Autodesk Fusion 360 part; units mm, degrees
sketch "Name Sign LED Holder Top" plane through (0, 0, 0) normal (0, 1, 0) x (1, 0, 0)
  line L0 (0.5771, -64.3591) -> (5.5771, -64.3591)
  line L1 (5.5771, -64.3591) -> (5.5771, -28.5209)
  line L2 (5.5771, -28.5209) -> (36.754, -15.7343)
  line L3 (36.754, -15.7343) -> (32.9594, -6.4822)
  line L4 (32.9594, -6.4822) -> (0.5771, -19.7631)
  line L5 (0.5771, -19.7631) -> (0.5771, -64.3591)
  line L6 (0.5771, -64.3591) -> (5.5771, -62.3085)
  line L7 (32.9594, -6.4822) -> (32.9594, -17.2905)
  dimension "d1" = 5
  dimension "d2" = 10
  dimension "d3" = 112.3
  dimension "d16" = 44.596
  dimension "d18" = 22.3
  dimension "d20" = 35
extrude "Extrude1" add sketch "Name Sign LED Holder Top" along normal blind 220 contours L1 L2 L4 L5 L6 L7
sketch "LED Grooves" plane through (0.5771, 0, 0) normal (-1, 0, 0) x (0, -1, 0)
  line L0 (0, 19.7631) -> (0, 64.3591)
  line L1 (-220, 64.3591) -> (-220, 19.7631)
  line L2 (-220, 19.7631) -> (0, 19.7631)
  line L3 (-215, 62.3591) -> (-5, 62.3591)
  line L4 (-5, 62.3591) -> (-5, 52.3591)
  line L5 (-5, 52.3591) -> (-215, 52.3591)
  line L6 (-215, 52.3591) -> (-215, 62.3591)
  line L7 (-215, 48.3591) -> (-5, 48.3591)
  line L8 (-5, 48.3591) -> (-5, 38.3591)
  line L9 (-5, 38.3591) -> (-215, 38.3591)
  line L10 (-215, 38.3591) -> (-215, 48.3591)
  line L11 (-5, 62.3591) -> (-15, 62.3591)
  line L12 (-15, 52.3591) -> (-5, 52.3591)
  line L13 (-5, 52.3591) -> (-5, 62.3591)
  line L14 (-5, 48.3591) -> (-15, 48.3591)
  line L15 (-15, 38.3591) -> (-5, 38.3591)
  line L16 (-5, 38.3591) -> (-5, 48.3591)
  line L17 (0, 64.3591) -> (-220, 64.3591)
  dimension "d6" = 210
  dimension "d7" = 210
  dimension "d8" = 5
  dimension "d9" = 5
  dimension "d12" = 10
  dimension "d13" = 10
  dimension "d22" = 4
  dimension "d30" = 2
extrude "Extrude2" cut sketch "LED Grooves" against normal blind 3 contours L3 L4 L5 L6 L11 L12 L13 | L7 L8 L9 L10 L14 L15 L16
sketch "Top LED Hole" plane through (3.5771, 0, 0) normal (-1, 0, 0) x (0, -1, 0)
  line L0 (-215, 52.3591) -> (-5, 52.3591)
  line L1 (-5, 52.3591) -> (-5, 62.3591)
  line L2 (-5, 62.3591) -> (-215, 62.3591)
  line L3 (-215, 62.3591) -> (-215, 52.3591)
  line L4 (-5, 62.3591) -> (-15, 62.3591)
  line L5 (-15, 62.3591) -> (-15, 52.3591)
  line L6 (-15, 52.3591) -> (-5, 52.3591)
  line L7 (-5, 52.3591) -> (-5, 62.3591)
  dimension "d33" = 10
  dimension "d34" = 10
sketch "Bottom LED Hole" plane through (3.5771, 0, 0) normal (-1, 0, 0) x (0, -1, 0)
  line L0 (-215, 38.3591) -> (-5, 38.3591)
  line L1 (-5, 38.3591) -> (-5, 48.3591)
  line L2 (-215, 48.3591) -> (-215, 38.3591)
  line L3 (-5, 48.3591) -> (-15, 48.3591)
  line L4 (-15, 48.3591) -> (-15, 38.3591)
  line L5 (-15, 38.3591) -> (-5, 38.3591)
  line L6 (-5, 38.3591) -> (-5, 48.3591)
  line L7 (-5, 48.3591) -> (-215, 48.3591)
  dimension "d26" = 10
  dimension "d27" = 10
extrude "Extrude3" cut sketch "Top LED Hole" sketch "Bottom LED Hole" against normal blind 2 contours L0 L1 L2 L4 L5 L6 L7 of sketch 2 contours L0 L1 L3 L4 L5 L6 L7
sketch "Magnet Holes" plane through (7.0215, 0, 17.1201) normal (-0.3795, 0, -0.9252) x (0, -1, 0)
  line L0 (0, -28.0347) -> (0, 6.9653)
  line L1 (0, 6.9653) -> (-220, 6.9653)
  line L2 (-220, 6.9653) -> (-220, -28.0347)
  line L3 (-220, -28.0347) -> (0, -28.0347)
  circle A0 centre (-210, -5.5347) radius 2.75
  dimension "d39" = 5.5
  dimension "d47" = 10
  dimension "d48" = 12.5
extrude "Extrude4" cut sketch "Magnet Holes" against normal blind 1.5 contours A0
pattern_linear "R-Pattern1" count 4 spacing 66.6667 along (0, -1, 0) count 2 spacing 15 along (0.9252, 0, -0.3795) of "Extrude4"
equation "d4 = 200 mm + 10 mm + 5 mm + 5 mm"
equation "d6 = 200 mm + 10 mm"
equation "d7 = 200 mm + 10 mm"
equation "d16 = 50 mm - 5.404 mm"
equation "magnet_hole_diameter = 5.5 mm"
equation "magnet_hole_depth = 1.5 mm"
equation "d39 = magnet_hole_diameter"
equation "d45 = magnet_pattern_height"
equation "magnet_hole_side_offset = 10 mm"
equation "d47 = magnet_hole_side_offset"
equation "d48 = vertical_part_width + magnet_hole_top_offset"
equation "magnet_hole_top_offset = 7.5 mm"
equation "magnet_pattern_length = 220.00 mm - 2 * ( magnet_hole_side_offset )"
equation "magnet_pattern_height = 35.00 mm - vertical_part_width - 2 * ( magnet_hole_top_offset )"
equation "vertical_part_width = 5.00 mm"
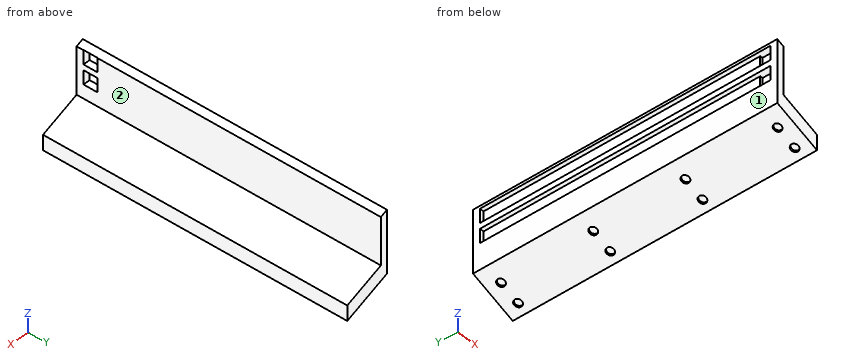
The listing builds one solid part. Answer for the finished solid, in the listing's coordinates (mm). Face numbers are marked on the shaded views. A direction names the side the tool comes from. Give positions to 0.01 mm unless a question says otherwise; leave off trailing zeros. Loops run counter-clockwise (first coordinate to the right, second up) from the corner with the lowest first, then second, coordinate; pieces in that order, holes last.
Item 1: A cutting plane is placed at C-C (y = 144). Give the vertices of the cut face in (x, z) (1 decimal).
Derived:
outline: (0.6, 19.8) - (9.7, 16) - (10.2, 17.4) - (15.2, 15.4) - (14.6, 14) - (23.6, 10.3) - (24.1, 11.7) - (29.1, 9.7) - (28.5, 8.3) - (33, 6.5) - (33, 17.3) - (5.6, 28.5) - (5.6, 62.3) - (0.6, 64.4) - (0.6, 62.4) - (3.6, 62.4) - (3.6, 52.4) - (0.6, 52.4) - (0.6, 48.4) - (3.6, 48.4) - (3.6, 38.4) - (0.6, 38.4) - close
Item 2: A cutting plane is placed at B-B (y = 31.5). Give the vertices of the cut face in (x, z), then the cut area to 3 significant figures.
Derived:
outline: (0.58, 19.76) - (32.96, 6.48) - (32.96, 17.29) - (5.58, 28.52) - (5.58, 62.31) - (0.58, 64.36) - (0.58, 62.36) - (3.58, 62.36) - (3.58, 52.36) - (0.58, 52.36) - (0.58, 48.36) - (3.58, 48.36) - (3.58, 38.36) - (0.58, 38.36) - close
area: 459 mm2
Item 3: A cutting plane is placed at D-D (x = 20). Give the vertices of the cut face in (y, z), then the cut area to 3 significant figures.
Derived:
outline: (0, 11.8) - (220, 11.8) - (220, 22.61) - (0, 22.61) - close
area: 2,380 mm2
Item 4: A tool of negligible diameter and unlimited length cuts with its end or side. For the marked faces 1 and 2, from which of +Z, -Z, +X, -X, +Y, -Y can it reach the whole face along a straight path? Write none if from no direction.
Derived:
face 1: +Z, -Z, -X, +Y, -Y
face 2: +Z, +X, +Y, -Y
Item 5: Each of these flat-tipped pins is pushed along its axis until it touches: pin 1 Ø6 at (y, z) = (141, 39) entering from +X; pin 2 Ø3 at (y, z) = (79, 59) entering from -X; pin 3 Ø6 at (x, y) = (24.5, 158.5) entering from -Z. Where does it stop, or does it pass through?
Derived:
pin 1: stops at x = 5.58
pin 2: stops at x = 3.58
pin 3: stops at z = 8.72
Item 6: Find the intervals of material crossed by line 1 along Z through (x, y) = (2, 32.5); line 2 along Y through (x, z) = (4, 59); line 3 along X through (y, z) = (36, 40.5), in increasing order.
Derived:
line 1: z = 19.18 to 38.36, 48.36 to 52.36, 62.36 to 63.78
line 2: y = 0 to 5, 15 to 220
line 3: x = 3.58 to 5.58
Item 7: A cutting plane is placed at A-A (z = 60). Give the vertices of the cut face in (x, y).
Derived:
outline: (0.58, 0) - (5.58, 0) - (5.58, 5) - (0.58, 5) - close; (0.58, 215) - (3.58, 215) - (3.58, 15) - (5.58, 15) - (5.58, 220) - (0.58, 220) - close
